from build123d import *

# Parameters (mm, degrees)
SKETCH1_R              = 14
BOSS_EXTRUDE1_DEPTH    = 2.5
M2_5_CLEARANCE_HOLE2_D = 2.5
CIRPATTERN1_COUNT      = 3
SKETCH7_W              = 1.025
SKETCH7_H              = 11.192782739


with BuildPart() as part:
    # Sketch1 → Boss-Extrude1 (new body, symmetric)
    with BuildSketch(Plane.XY):
        Circle(SKETCH1_R)
        with BuildLine():
            Line((-1.5875, 2.807217261), (1.5875, 2.807217261))
            ThreePointArc((1.5875, 2.807217261), (0, -3.225), (-1.5875, 2.807217261))
        make_face(mode=Mode.SUBTRACT)
    extrude(amount=BOSS_EXTRUDE1_DEPTH, both=True)

    # M2.5 Clearance Hole2 (through all)
    with Locations(Plane.XY.offset(2.5)):
        with Locations((0, -10)):
            m2_5_clearance_hole2 = Hole(M2_5_CLEARANCE_HOLE2_D / 2)

    # CirPattern1: M2.5 Clearance Hole2 ×3 about axis
    cirpattern1_axis = Axis((0, 0, 0), (0, 0, 1))
    for i in range(1, CIRPATTERN1_COUNT):
        add(m2_5_clearance_hole2.rotate(cirpattern1_axis, i * 360 / CIRPATTERN1_COUNT), mode=Mode.SUBTRACT)

    # Sketch7 → M2.5x0.45 Tapped Hole1 (revolve, cut)
    with BuildSketch(Plane(origin=(0, 2.807217261, 0), x_dir=(0, 0, -1), z_dir=(1, 0, 0))):
        with Locations((0.5125, 5.59639137)):
            Rectangle(SKETCH7_W, SKETCH7_H)
    revolve(axis=Axis((0, -3.542782739, 0), (0, 1, 0)), mode=Mode.SUBTRACT)


solid = part.part
Source: CAD feature listing. Evaluate the final solid. Frame: model axes, mm. A direction names the side the tool comes from. Coordinates: 2 decimals unless noted, no trailing zeros. Write each loop counter-clockwise with the first axis right and the second up, starting at its lowest first coordinate (ties: lowest second). Pieces come first, ordered by that corner, then holes. Notation, with made-up numbers: M 30.25,17 L 49.25,17 A23 ccw 49.25,32 Z; hole C 47.25,62.25 d9. An arc over 180 degrees is marked long. Use a Markdown table: item, result.
1) First-contact query: pin 1 Ø3 at (x, z) = (-7, 1.5) entering from +Y; pin 2 Ø3 at (y, z) = (8, 0) entering from -X; pin 3 Ø1 at (x, z) = (4, -1.5) entering from +Y. Flat tips, straight axial feed; report the tip coordinate or a pass-through.
Conclusion:
| item | result |
|---|---|
| pin 1 | stops at y = 12.87 |
| pin 2 | stops at x = -12.4 |
| pin 3 | stops at y = 13.56 |
2) Mould query, pull axis X, two halves, no side actions, for faces 1 (the cylindrical face through (-0.672, -8.946, -0.035)), 2 (the cylindrical face through (12.932, -5.362, 0.035)), 3 (the flat face through (0, 3, -2.5)). Classes: pulls with the +X half, pulls with the -X half, needs draft (parallel to the pull), parting line crosses it, or undercut.
Conclusion:
| item | result |
|---|---|
| face 1 | undercut |
| face 2 | parting line crosses it |
| face 3 | needs draft |
3) Section A-A, the plane y = 0. Output: boundary loops of the cut face in (x, z) (3 decimals).
Conclusion:
| item | result |
|---|---|
| outline | M -14,-2.5 L -3.225,-2.5 L -3.225,2.5 L -14,2.5 Z; M 3.225,-2.5 L 14,-2.5 L 14,2.5 L 3.225,2.5 Z |
4) Ray query, L1, parallel to Y at x = 0, z = 0.3 (3 decimals); L2, parallel to Z at x = 0, y = 9 (3 decimals); L3, parallel to Y at x = 1.75, z = 0.95. Return the intervals inside material, ascending.
Conclusion:
| item | result |
|---|---|
| L1 | y = -14 to -11.25, -8.75 to -3.225 |
| L2 | z = -2.5 to -1.025, 1.025 to 2.5 |
| L3 | y = -13.89 to -2.71, 2.71 to 13.89 |
5) Section D-D, the plane x = 12.25. Output: boundary loops of the cut face in (y, z), then the cut area to 3 significant figures.
Conclusion:
| item | result |
|---|---|
| outline | M -6.78,-2.5 L 6.78,-2.5 L 6.78,2.5 L -6.78,2.5 Z |
| area | 67.8 mm^2 |
6) Reachability of faces 4 (the flat face through (0.33, 2.807, 1.15)), 5 (the flat face through (0, 3, 2.5)), 6 (the cylindrical face through (-1.016, 8.482, 0.133)) from +Z, -Z, +X, -X, +Y, -Y: full face, straight path, thin tool, end or side. Return the list, or none.
Conclusion:
| item | result |
|---|---|
| face 4 | +Z, -Z |
| face 5 | +Z, +X, -X, +Y, -Y |
| face 6 | +Y |
7) Section B-B, the plane z = 0.7. Give the number of separate pieces and of enclosed holes in the cut face, then the cut area to 3 significant figures.
Conclusion:
| item | result |
|---|---|
| separate pieces | 1 |
| enclosed holes | 3 |
| area | 552 mm^2 |
8) Section C-C, the plane y = 5. Output: boundary loops of the cut face in (x, z) (3 decimals).
Conclusion:
| item | result |
|---|---|
| outline | M -13.077,-2.5 L -9.91,-2.5 L -9.91,2.5 L -13.077,2.5 Z; M -7.41,-2.5 L 7.41,-2.5 L 7.41,2.5 L -7.41,2.5 Z; M 9.91,-2.5 L 13.077,-2.5 L 13.077,2.5 L 9.91,2.5 Z; hole C 0,0 d2.05 |
